Design review of the part shown in the three views and the two pictorial views. Dimensions are in mm from the part's minimum x, y and z. Coordinates: 2 decimals unless noted, no trailing zeros. Order: outer loops, then holes, each group sorted by start corner. A loop starts at its lowest first (then second) coordinate and runs counter-clockwise, first axis right, second up. Notation, with made-up numbers: (20, 25.5) - (45, 25.5) arc R26 ccw to (45, 49.5) - close; hole circle Ø7 at (37.5, -27.5). An arc over 180 degrees is marked (long way). One line per item, written item: value. Start each with the question number.
(1) Consider section D-D on z = 5. Write out the cut boundary in (x, y).
(2) Consider section B-B on x = 10. Write out the cut boundary in (y, z), then the cut area to 3 significant figures.
(3) To check wall thickness, follow line 1 along Z through (x, y) = (10, 11); line 2 along Z through (x, y) = (10, 16.25); line 3 along Z through (x, y) = (10, 18.75). State the ranges of each line that lie inside material, in increasing order.
(4) Mouldability with a two-part tool opening along X and no side actions: class the marked faces 1, 2 and 3 as released by +X, released by -X, zero draft, split by the parting line, or undercut.
(5) Consider section C-C on y = 20.25. Write out the cut boundary in (x, z).
(6) Consider section A-A on z = 36. Write out the cut boundary in (x, y), then the cut area to 3 significant figures.
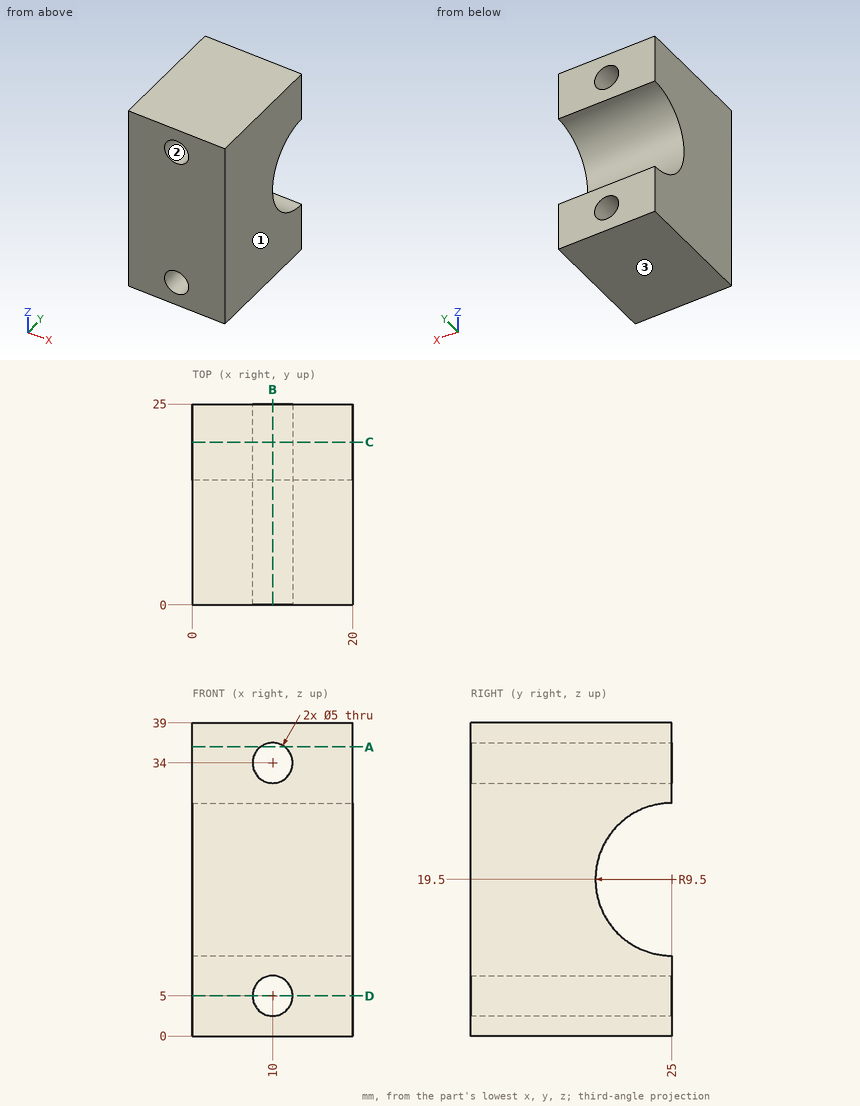
Geometry check:
1. outline: (0, 0) - (7.5, 0) - (7.5, 25) - (0, 25) - close; (12.5, 0) - (20, 0) - (20, 25) - (12.5, 25) - close
2. outline: (0, 0) - (25, 0) - (25, 2.5) - (0, 2.5) - close; (0, 7.5) - (25, 7.5) - (25, 10) arc R9.5 cw to (25, 29) - (25, 31.5) - (0, 31.5) - close; (0, 36.5) - (25, 36.5) - (25, 39) - (0, 39) - close
2. area: 583 mm^2
3. line 1: z = 0 to 2.5, 7.5 to 31.5, 36.5 to 39
3. line 2: z = 0 to 2.5, 7.5 to 15.8, 23.2 to 31.5, 36.5 to 39
3. line 3: z = 0 to 2.5, 7.5 to 12.35, 26.65 to 31.5, 36.5 to 39
4. face 1: released by +X
4. face 2: undercut
4. face 3: zero draft
5. outline: (0, 0) - (20, 0) - (20, 11.27) - (0, 11.27) - close; (0, 27.73) - (20, 27.73) - (20, 39) - (0, 39) - close; hole circle Ø5 at (10, 5); hole circle Ø5 at (10, 34)
6. outline: (0, 0) - (8.5, 0) - (8.5, 25) - (0, 25) - close; (11.5, 0) - (20, 0) - (20, 25) - (11.5, 25) - close
6. area: 425 mm^2
